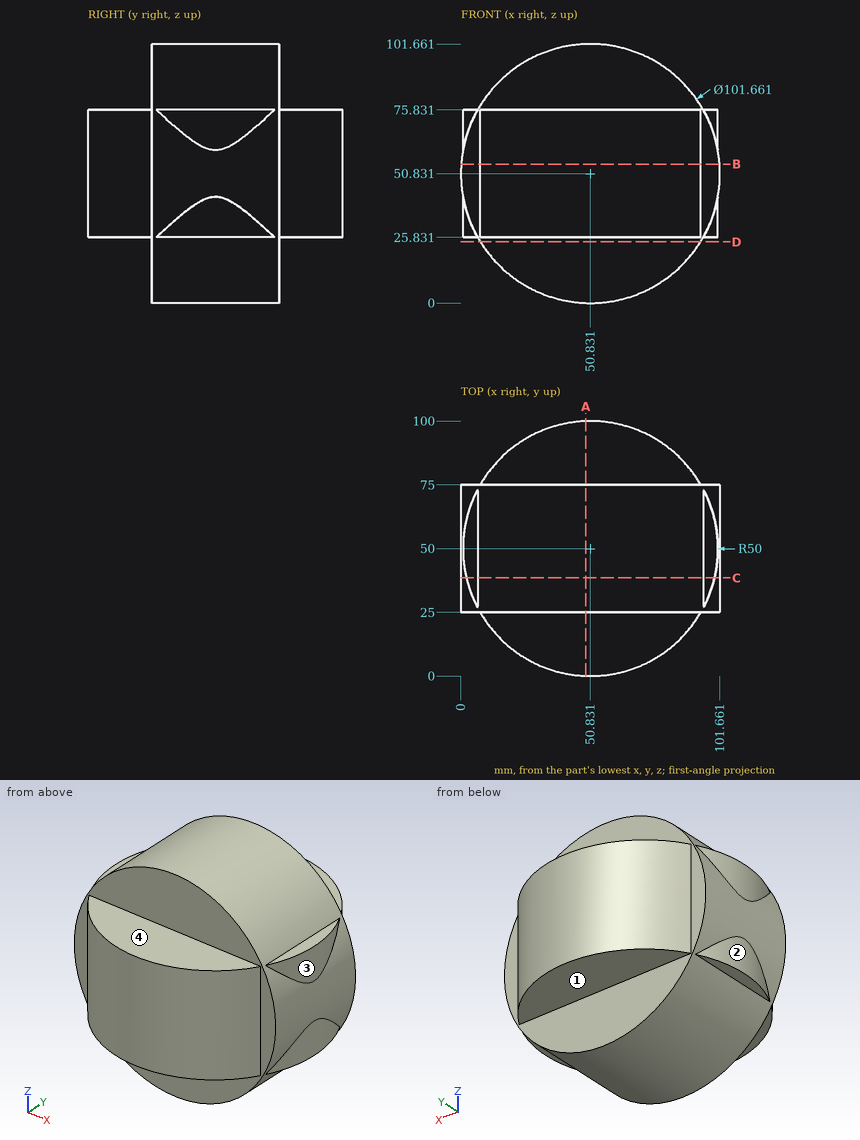
For this review, use the dimensioned drawing (mm, ordinates from the lowest corner) and the shaded views. A direction names the side the tool comes from. Round coordinates to 2 decimals unless told otherwise and drop trailing zeros. Loops run counter-clockwise (first coordinate to the right, second up) from the corner with the lowest first, then second, coordinate; pieces in that order, holes last. Notation, with made-up numbers: M -37.5,75 L -23.5,75 A11 cw -23.5,90 Z; hole C 47,39.25 d4. An arc over 180 degrees is marked long. Answer as a JSON object with one key per item and string values.
(1) Take a section at B-B on z = 54.5. Give the boundary of the cut face in (x, y).
Resolved:
{"outline": "M 0.13,25 L 7.53,25 A50 ccw 94.13,25 L 101.53,25 L 101.53,75 L 94.13,75 A50 ccw 7.53,75 L 0.13,75 Z"}
(2) Take a section at D-D on z = 24. Give the boundary of the cut face in (x, y), and give its area (3 significant figures).
Resolved:
{"outline": "M 7.66,25 L 94,25 L 94,75 L 7.66,75 Z", "area": "4,320 mm²"}
(3) Tool access review of the marked faces 1, 2, 3 and 4: name each direction out of +Z, -Z, +X, -X, +Y, -Y from which nothing blocks a thin tool from reaching the whole face with its end or side.
Resolved:
{"face 1": "-Z, +X, -X, +Y", "face 2": "-Z, -X", "face 3": "+Z, +X", "face 4": "+Z, +X, -X, -Y"}
(4) Take a section at C-C on y = 38.5. Give the boundary of the cut face in (x, z), and give its area (3 significant figures).
Resolved:
{"outline": "M 2.17,25.83 L 6.57,25.83 A50.83 ccw 95.09,25.83 L 99.49,25.83 L 99.49,36.13 A50.83 ccw 99.49,65.53 L 99.49,75.83 L 95.09,75.83 A50.83 ccw 6.57,75.83 L 2.17,75.83 L 2.17,65.53 A50.83 ccw 2.17,36.13 Z", "area": "8,200 mm²"}
(5) Clearance check with flat-ended pins moving along their axes: P1, Ø8, axis at y = 11.5, z = 38.5, coming from the -X side; P2, Ø4, axis at x = 72, z = 18, coming from the -Y side; P3, Ø4, axis at y = 53, z = 60.5, coming from the -X side. State where each tip first meets the part, or that it passes through.
Resolved:
{"P1": "x = 14.64", "P2": "y = 25", "P3": "x = 0.58"}
(6) To check wall thickness, follow line 1 along Z through (x, y) = (16.5, 78); line 2 along Y through (x, z) = (42, 19); line 3 along Y through (x, z) = (64.5, 49) (1 decimal). State the ranges of each line that lie inside material, in increasing order.
Resolved:
{"line 1": "25.83 to 75.83", "line 2": "25 to 75", "line 3": "1.9 to 98.1"}
(7) Take a section at A-A on x = 49. Give the boundary of the cut face in (y, z).
Resolved:
{"outline": "M 0.03,25.83 L 25,25.83 L 25,0.03 L 75,0.03 L 75,25.83 L 99.97,25.83 L 99.97,75.83 L 75,75.83 L 75,101.63 L 25,101.63 L 25,75.83 L 0.03,75.83 Z"}
